Work out the finished part from the listing and answer in its coordinate system (mm). A direction names the side the tool comes from. Round coordinates to 2 decimals unless told otherwise and drop trailing zeros. Order: outer loops, then holes, each group sorted by start corner. A loop starts at its lowest first (then second) coordinate and runs counter-clockwise, first axis right, second up. Notation, with made-up numbers: (72.25, 45.5) -> (99.25, 45.5) arc R9 ccw to (99.25, 55.5) -> close; hole circle Ø4 at (51, 79). An arc over 180 degrees is marked (long way). Use a Markdown table: item, result. Add a question column.
Item 1: For a pull along X with two mould halves and no side action, classify faces 1 (the flat face through (-2, 2, 0)), 2 (the flat face through (7.5, 0, 12)), 3 (the cylindrical face through (0.401, -1.806, 10.353)) as +X half, -X half, draft (parallel to the pull), parting line (faces both ways), or undercut.
Item 2: Flat-ended cylindrical pins translate along their axes: P1, Ø5, axis at x = -5.5, y = 5.5, coming from the +Z side; P2, Ø3.5, axis at x = 0.5, y = -1, coming from the +Z side. Find the tip coordinate at first contact, or state that the pin passes through.
Item 3: A cutting plane is placed at C-C, the plane y = -4.25. Determine the outline of the cut face in (x, z), plus the area to 3 significant figures.
Item 4: A cutting plane is placed at D-D, the plane z = 6. Determine the outline of the cut face in (x, y), plus the area to 3 significant figures.
Item 5: A tool of negligible diameter and unlimited length cuts with its end or side. For faces 4 (the flat face through (0, -7.5, 22)), 5 (the flat face through (-2, 3, 25)), 6 (the flat face through (-7.5, 0, 14)), 7 (the cylindrical face through (0, -4, 33)), 8 (the cylindrical face through (-0.45, 3.42, 23.03)), from which of +Z, -Z, +X, -X, +Y, -Y can it reach the whole face along a straight path? Write none if from no direction.
Item 6: A cutting plane is placed at A-A, the plane x = 0. Give the number of separate pieces and of enclosed holes in the cut face, plus the area to 3 significant figures.
Item 7: Find the intervals of material crossed by L1, parallel to X at y = -4.2, z = 35; L2, parallel to Z at x = 0, y = 3.75; L3, parallel to Y at x = -2, z = 27.5, in increasing order. Write a range as [from, to].
Item 8: A cutting plane is placed at B-B, the plane y = 0. Determine the outline of the cut face in (x, z), plus the area to 3 significant figures.
from build123d import *

# Parameters (mm, degrees)
F1_DEPTH       = 25
F3_D           = 3.7
F3_CBORE_D     = 6.9
F3_CBORE_DEPTH = 4
F5_DEPTH       = 4
F7_DEPTH       = 4
F9_D           = 4
F9_DEPTH       = 4
F9_CSINK_D     = 8.2
F9_CSINK_ANGLE = 90
F11_D          = 3.3
F11_DEPTH      = 4


with BuildPart() as f1:
    # F0 (on Top) → F1 (new body)
    with BuildSketch(Plane.XY):
        Polygon((7.5, -7.5), (7.5, 0), (7.5, 7.5), (-7.5, 7.5), (-7.5, -7.5), align=None)
    extrude(amount=F1_DEPTH)

    # F3 (through all)
    with Locations(Plane.XY.offset(25)):
        with Locations((0, 0)):
            CounterBoreHole(F3_D / 2, F3_CBORE_D / 2, F3_CBORE_DEPTH)

    # F4 (on face) → F5 (join)
    with BuildSketch(Plane(origin=(0, 7.5, 0), x_dir=(-1, 0, 0), z_dir=(0, 1, 0))):
        with BuildLine():
            Line((-7.5, 25), (7.5, 25))
            Line((7.5, 25), (7.5, 35))
            ThreePointArc((7.5, 35), (6, 30.5), (2.1, 27.8))
            Line((2.1, 27.8), (-7.5, 25))
        make_face()
        with BuildLine():
            ThreePointArc((2.1, 27.8), (6, 30.5), (7.5, 35))
            ThreePointArc((7.5, 35), (-6, 39.5), (2.1, 27.8))
        make_face()
    extrude(amount=-F5_DEPTH)

    # F6 (on face) → F7 (join)
    with BuildSketch(Plane.XZ.offset(7.5)):
        with BuildLine():
            ThreePointArc((7.5, 35), (0, 42.5), (-7.5, 35))
            ThreePointArc((-7.5, 35), (-6, 30.5), (-2.1, 27.8))
            ThreePointArc((-2.1, 27.8), (4.5, 29), (7.5, 35))
        make_face()
        with BuildLine():
            Line((-7.5, 35), (-7.5, 25))
            Line((-7.5, 25), (7.5, 25))
            Line((7.5, 25), (-2.1, 27.8))
            ThreePointArc((-2.1, 27.8), (-6, 30.5), (-7.5, 35))
        make_face()
    extrude(amount=-F7_DEPTH)

    # F9
    with Locations(Plane.XZ.offset(7.5)):
        with Locations((0, 35)):
            CounterSinkHole(F9_D / 2, F9_CSINK_D / 2, depth=F9_DEPTH, counter_sink_angle=F9_CSINK_ANGLE)

    # F11
    with Locations(Plane(origin=(0, 7.5, 0), x_dir=(-1, 0, 0), z_dir=(0, 1, 0))):
        with Locations((0, 35)):
            Hole(F11_D / 2, depth=F11_DEPTH)


solid = f1.part
Reported:
| question | item | result |
|---|---|---|
| 1 | face 1 | draft |
| 1 | face 2 | +X half |
| 1 | face 3 | undercut |
| 2 | P1 | z = 41.87 |
| 2 | P2 | z = 21 |
| 3 | outline | (-7.5, 0) -> (7.5, 0) -> (7.5, 25) -> (-2.1, 27.8) arc R7.5 ccw (long way) to (-7.5, 35) -> close; hole circle Ø4 at (0, 35) |
| 3 | area | 578 mm² |
| 4 | outline | (-7.5, -7.5) -> (7.5, -7.5) -> (7.5, 7.5) -> (-7.5, 7.5) -> close; hole circle Ø3.7 at (0, 0) |
| 4 | area | 214 mm² |
| 5 | face 4 | +Z, -Z, +X, -X, -Y |
| 5 | face 5 | +Z, +X, -X |
| 5 | face 6 | +Z, -Z, -X, +Y, -Y |
| 5 | face 7 | -Y |
| 5 | face 8 | +Z |
| 6 | separate pieces | 6 |
| 6 | enclosed holes | 0 |
| 6 | area | 374 mm² |
| 7 | L1 | [-7.5, -2], [2, 7.5] |
| 7 | L2 | [0, 27.19], [27.5, 33.35], [36.65, 42.5] |
| 7 | L3 | [-7.5, -3.5], [3.5, 7.5] |
| 8 | outline | (-7.5, 0) -> (-1.85, 0) -> (-1.85, 21) -> (-3.45, 21) -> (-3.45, 25) -> (-7.5, 25) -> close; (1.85, 0) -> (7.5, 0) -> (7.5, 25) -> (3.45, 25) -> (3.45, 21) -> (1.85, 21) -> close |
| 8 | area | 270 mm² |
